Can you work these out from the model? Positions are in its coordinate system, mm. Face numbers are marked on the shaded views. A direction names the side the tool comes from. Round coordinates to 2 decimals unless told otherwise and drop trailing zeros. Write each loop counter-clockwise with the first axis right and the second up, starting at its lowest first coordinate (ties: lowest second). Pieces come first, ordered by that corner, then holes. Notation, with made-up numbers: M -16.75,30.25 L 0.25,30.25 A18 ccw 0.25,49.25 Z; hole C -2.5,-12.75 d4. An arc over 180 degrees is marked long. Answer in a Markdown table with one row per item. Add a question column.
(1) If I drill on probe 1 along Z at (x, y) = (280.5, 31); probe 2 along X at (y, z) = (44, -436); probe 3 along X at (y, z) = (3, -218.5), over which ranges is the centre line in solid material (lowest first)?
(2) I'm going to push flat-ended pins straight in: pin 1 (4 mm diameter, centred on x = 343, z = -304, fed in from +Y); pin 2 (4 mm diameter, centred on x = 211, z = -311, fed in from +Y). Where does each tip first touch, or does it pass through?
(3) Suppose I cut it at C-C, the plane z = -486.5. Write out the boundary of the cut face in (x, y).
(4) For the marked faces 1 and 2, which set-ups out of +Z, -Z, +X, -X, +Y, -Y let a thin tool reach every point of the face, with its end or its side?
(5) Suppose I cut it at B-B, the plane x = 41.5. Write out the boundary of the cut face in (y, z).
(6) If we mould it in two halves opening along Z, with no side actions, what happens to the marked faces 3, 4 and 5? For each: released by +Z, released by -Z, zero draft, split by the parting line, or undercut.
(7) Suppose I cut it at A-A, the plane y = 17.5. Write out the boundary of the cut face in (x, z).
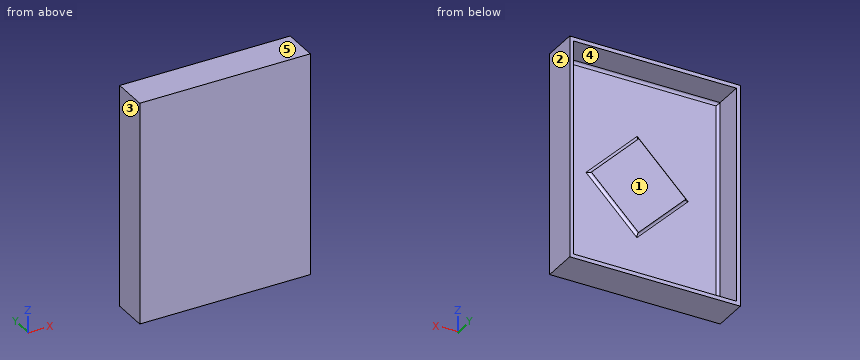
from build123d import *

# Parameters (mm, degrees)
SKETCH2_W           = 439.1
SKETCH2_H           = 572.45
SKETCH2_W_2         = 419.1
SKETCH2_H_2         = 552.45
BOSS_EXTRUDE1_DEPTH = 80.42
BOSS_EXTRUDE2_DEPTH = 7.16
SKETCH4_W           = 439.1
SKETCH4_H           = 572.45
BOSS_EXTRUDE3_DEPTH = 10
FILLET1_R           = 7


with BuildPart() as part:
    # Sketch2 → Boss-Extrude1 (new body)
    with BuildSketch(Plane(origin=(0, 0, 0), x_dir=(1, 0, 0), z_dir=(0, 1, 0))):
        with Locations((209.55, 276.225)):
            Rectangle(SKETCH2_W, SKETCH2_H)
        with Locations((209.55, 276.225)):
            Rectangle(SKETCH2_W_2, SKETCH2_H_2, mode=Mode.SUBTRACT)
    extrude(amount=BOSS_EXTRUDE1_DEPTH)



with BuildPart() as body_2:
    # Sketch3 → Boss-Extrude2 (new body)
    with BuildSketch(Plane(origin=(0, 0, 0), x_dir=(1, 0, 0), z_dir=(0, 1, 0))):
        Polygon((88.316542366, 276.225), (209.55, 154.991542366), (331.455559866, 276.897102232), (210.222102232, 398.130559866), align=None)
    extrude(amount=BOSS_EXTRUDE2_DEPTH)


with BuildPart() as part_1:
    add(part.part)

    add(body_2.part)  # Boss-Extrude3 merges body 2
    # Sketch4 → Boss-Extrude3 (add)
    with BuildSketch(Plane(origin=(0, 0, 0), x_dir=(1, 0, 0), z_dir=(0, 1, 0))):
        with Locations((209.55, 276.225)):
            Rectangle(SKETCH4_W, SKETCH4_H)
    extrude(amount=-BOSS_EXTRUDE3_DEPTH)

    # Fillet1
    fillet1_edges = [part_1.edges().sort_by_distance(p)[0] for p in [
        (0, 0, -276.225),
        (209.55, 0, 0),
        (419.1, 0, -276.225),
        (209.55, 0, -552.45),
        (149.269322299, 0, -337.177779933),
        (148.933271183, 0, -215.608271183),
        (270.502779933, 0, -215.944322299),
        (270.838831049, 0, -337.513831049),
    ]]
    fillet(fillet1_edges, radius=FILLET1_R)


solid = part_1.part
Calculated:
| question | item | result |
|---|---|---|
| 1 | probe 1 | -562.45 to -552.45, 0 to 10 |
| 1 | probe 2 | -10 to 0, 419.1 to 429.1 |
| 1 | probe 3 | -10 to 1.26, 144.27 to 274.83, 417.84 to 429.1 |
| 2 | pin 1 | y = 0 |
| 2 | pin 2 | y = 7.16 |
| 3 | outline | M -10,-10 L 429.1,-10 L 429.1,80.42 L 419.1,80.42 L 419.1,7 A7 cw 412.1,0 L 7,0 A7 cw 0,7 L 0,80.42 L -10,80.42 Z |
| 4 | face 1 | +Y |
| 4 | face 2 | +Z, -Z, +X, +Y, -Y |
| 5 | outline | M -10,-562.45 L 80.42,-562.45 L 80.42,-552.45 L 7,-552.45 A7 cw 0,-545.45 L 0,-7 A7 cw 7,0 L 80.42,0 L 80.42,10 L -10,10 Z |
| 6 | face 3 | zero draft |
| 6 | face 4 | undercut |
| 6 | face 5 | released by +Z |
| 7 | outline | M -10,-562.45 L 429.1,-562.45 L 429.1,10 L -10,10 Z; hole M 0,-552.45 L 419.1,-552.45 L 419.1,0 L 0,0 Z |
